Model file for the job. Use its own axes, mm. Face numbers are marked on the shaded views. Round coordinates to 2 decimals unless told otherwise and drop trailing zeros. Order: outer loops, then holes, each group sorted by start corner. A loop starts at its lowest first (then second) coordinate and runs counter-clockwise, first axis right, second up. Notation, with made-up numbers: M 75.5,-3.75 L 81.5,-3.75 A24 ccw 81.5,32.25 Z; hole C 35.5,-40 d9. An arc over 180 degrees is marked long. Return JSON: item names as keys, results as strings. Group by question number.
Item 1: Slice it at C-C on y = 0. Write the cut outline in (x, z).
Item 2: Pull direction X, two halves, no side cores. Call the marked faces 1, 2 and 3: pulls with the +X half, pulls with the -X half, needs draft (parallel to the pull), parting line crosses it, or undercut.
Item 3: Probe line 1 along Y through (x, z) = (19.05, 15.75) (3 decimals); line 2 along Y through (x, z) = (0, 7); line 3 along Y through (x, z) = (-21, 16). List the from-to ranges inside material, lowest first.
Item 4: Slice it at D-D on x = 11.5. Write the cut outline in (y, z), then the cut area to 3 significant figures.
Item 5: Pin check, flat tip, straight feed: pin 1 Ø8.5 at (x, y) = (19.05, -19.05) entering from +Z. Stop position of the tip, or through.
Item 6: Slice it at A-A on y = -19.05. Write the cut outline in (x, z) (3 decimals), then the cut area to 3 significant figures.
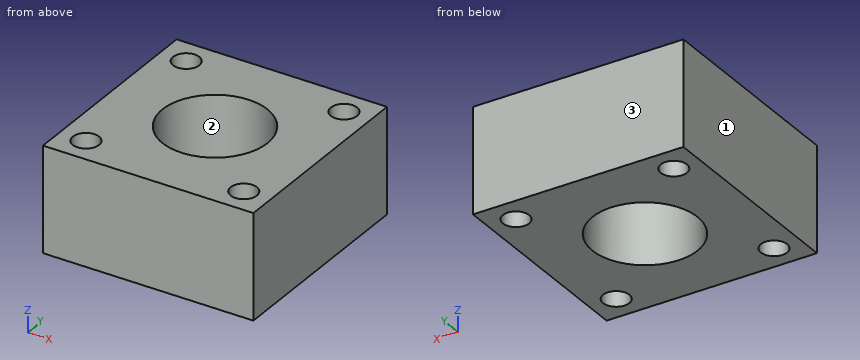
from build123d import *

# Parameters (mm, degrees)
SKETCH4_W           = 50.8
SKETCH4_H           = 50.8
BOSS_EXTRUDE2_DEPTH = 25.4
SKETCH5_R           = 3.175
SKETCH5_R_2         = 12.7
CUT_EXTRUDE5_DEPTH  = 25.4


with BuildPart() as part:
    # Sketch4 → Boss-Extrude2 (new body)
    with BuildSketch(Plane.XY):
        Rectangle(SKETCH4_W, SKETCH4_H)
    extrude(amount=BOSS_EXTRUDE2_DEPTH)

    # Sketch5 → Cut-Extrude5 (cut)
    with BuildSketch(Plane.XY.offset(25.4)):
        with Locations((19.05, 19.05)):
            Circle(SKETCH5_R)
        Circle(SKETCH5_R_2)
        with Locations((-19.05, 19.05)):
            Circle(SKETCH5_R)
        with Locations((19.05, -19.05)):
            Circle(SKETCH5_R)
        with Locations((-19.05, -19.05)):
            Circle(SKETCH5_R)
    extrude(amount=-CUT_EXTRUDE5_DEPTH, mode=Mode.SUBTRACT)


solid = part.part
Output values:
{
 "1": {"outline": "M -25.4,0 L -12.7,0 L -12.7,25.4 L -25.4,25.4 Z; M 12.7,0 L 25.4,0 L 25.4,25.4 L 12.7,25.4 Z"},
 "2": {"face 1": "pulls with the -X half", "face 2": "undercut", "face 3": "needs draft"},
 "3": {"line 1": "-25.4 to -22.225, -15.875 to 15.875, 22.225 to 25.4", "line 2": "-25.4 to -12.7, 12.7 to 25.4", "line 3": "-25.4 to -21.56, -16.54 to 16.54, 21.56 to 25.4"},
 "4": {"outline": "M -25.4,0 L -5.39,0 L -5.39,25.4 L -25.4,25.4 Z; M 5.39,0 L 25.4,0 L 25.4,25.4 L 5.39,25.4 Z", "area": "1,020 mm²"},
 "5": {"pin 1": "z = 25.4"},
 "6": {"outline": "M -25.4,0 L -22.225,0 L -22.225,25.4 L -25.4,25.4 Z; M -15.875,0 L 15.875,0 L 15.875,25.4 L -15.875,25.4 Z; M 22.225,0 L 25.4,0 L 25.4,25.4 L 22.225,25.4 Z", "area": "968 mm²"}
}
